Input: part model. Units: mm. Frame: model coordinates. Round coordinates to 2 decimals unless told otherwise and drop trailing zeros. Loops run counter-clockwise (first coordinate to the right, second up) from the corner with the lowest first, then second, coordinate; pieces in that order, holes last. Notation, with made-up numbers: (3, -7) -> (47, -7) arc R13 ccw to (47, 11) -> close; hole circle Ø5 at (22, 51.5). An arc over 180 degrees is marked (long way). Answer as a JSON object with one key per item and string values.
```python
from build123d import *

# Parameters (mm, degrees)
F0_R     = 5.05
F1_DEPTH = 10.8
F2_R     = 5.05
F3_R     = 3.2
F4_DEPTH = 9.1
F5_R     = 0.3


with BuildPart() as f1:
    # F0 (on Top) → F1 (new body)
    with BuildSketch(Plane.XY):
        Circle(F0_R)
    extrude(amount=F1_DEPTH)

    # F2
    f2_edges = [f1.edges().sort_by_distance(p)[0] for p in [
        (-5.05, 0, 10.8),
    ]]
    fillet(f2_edges, radius=F2_R)

    # F3 (on face) → F4 (cut)
    with BuildSketch(Plane(origin=(0, 0, 0), x_dir=(1, 0, 0), z_dir=(0, 0, -1))):
        Circle(F3_R)
    extrude(amount=-F4_DEPTH, mode=Mode.SUBTRACT)

    # F5
    f5_edges = [f1.edges().sort_by_distance(p)[0] for p in [
        (-3.2, 0, 9.1),
    ]]
    fillet(f5_edges, radius=F5_R)


solid = f1.part
```
1) Draft query along X for faces 1 (the face through (4.817, 1.517, 2.835)), 2 (the face through (1.1, -3.3, 0)), 3 (the face through (0, 0, 9.1)). Return one class per face: +X half, -X half, draft (parallel to the pull), parting line (faces both ways), or undercut.
Output:
{"face 1": "parting line", "face 2": "draft", "face 3": "undercut"}
2) Section B-B, the plane z = 6.75. Output: boundary loops of the cut face in (x, y), plus the area to 3 significant figures.
Output:
{"outline": "circle Ø9.9 at (0, 0); hole circle Ø6.4 at (0, 0)", "area": "44.8 mm^2"}
3) Ray query, probe 1 along Y at (x, z) = (0, 5.5); probe 2 along Y at (x, z) = (0, 7.25); probe 3 along X at (y, z) = (-2.5, 2.75). Return the intervals inside material, ascending.
Output:
{"probe 1": "y = -5.05 to -3.2, 3.2 to 5.05", "probe 2": "y = -4.82 to -3.2, 3.2 to 4.82", "probe 3": "x = -4.39 to -2, 2 to 4.39"}
4) Section A-A, the plane x = 0. Output: boundary loops of the cut face in (y, z), plus the area to 3 significant figures.
Output:
{"outline": "(-5.05, 0) -> (-3.2, 0) -> (-3.2, 8.8) arc R0.3 cw to (-2.9, 9.1) -> (2.9, 9.1) arc R0.3 cw to (3.2, 8.8) -> (3.2, 0) -> (5.05, 0) -> (5.05, 5.75) arc R5.05 ccw to (-5.05, 5.75) -> close", "area": "39.9 mm^2"}
5) Section D-D, the plane z = 1. Output: boundary loops of the cut face in (x, y), plus the area to 3 significant figures.
Output:
{"outline": "circle Ø10.1 at (0, 0); hole circle Ø6.4 at (0, 0)", "area": "47.9 mm^2"}
6) Contact query for flat-ended pins moving along their axis: P1, Ø1, axis at y = -2.5, z = 1.5, coming from the +X side; P2, Ø2, axis at x = 0.5, y = -3.5, coming from the +Z side; P3, Ø1.5, axis at x = -3.5, z = 6.5, coming from the +Y side. Output: stop coordinate, or through.
Output:
{"P1": "stops at x = 4.64", "P2": "stops at z = 10.12", "P3": "stops at y = 4.18"}
